```python
from build123d import *

# Parameters (mm, degrees)
F0_W      = 44.656470418
F0_H      = 33.8078811765
F1_DEPTH  = 16
F2_DEPTH  = 796
F3_DEPTH  = 196
F4_W      = 68.9578056335
F4_H      = 493.6993122101
F5_DEPTH  = 7
F6_DEPTH  = 9.7
F7_DEPTH  = 99.33
F8_DEPTH  = 99.33
F9_DEPTH  = 17.34
F10_DEPTH = 102.97
F11_W     = 35.2807044983
F11_H     = 492.0964837074
F12_DEPTH = 7
F13_DEPTH = 37.27
F14_DEPTH = 6.58
F15_DEPTH = 106.63
F16_DEPTH = 5.87
F17_DEPTH = 200
F18_DEPTH = 200
F19_DEPTH = 200
F20_DEPTH = 200
F21_DEPTH = 200
F22_DEPTH = 200
F23_DEPTH = 400
F24_DEPTH = 400
F25_DEPTH = 400
F26_DEPTH = 400
F27_DEPTH = 400
F28_DEPTH = 400
F29_DEPTH = 400
F30_DEPTH = 400
F31_DEPTH = 400
F32_DEPTH = 1000
F33_DEPTH = 1000
F34_DEPTH = 1000
F35_DEPTH = 1000
F36_DEPTH = 1000
F37_DEPTH = 1000
F38_R     = 3


with BuildPart() as f1:
    # F0 (on Front) → F1 (new body)
    with BuildSketch(Plane.XZ):
        with Locations((22.328235209, 16.9039405882)):
            Rectangle(F0_W, F0_H)
    extrude(amount=F1_DEPTH)

    # F2 (add): a face of the model
    f2_faces = [f1.faces().sort_by_distance(p)[0] for p in [
        (22.328235209, -8, 0),
    ]]
    extrude(f2_faces, amount=-F2_DEPTH)

    # F3 (add): a face of the model
    f3_faces = [f1.faces().sort_by_distance(p)[0] for p in [
        (0, -8, 398),
    ]]
    extrude(f3_faces, amount=-F3_DEPTH)

    # F4 (on face) → F5 (cut)
    with BuildSketch(Plane.XZ.offset(16)):
        with Locations((94.1769480705, 399.8196721077)):
            Rectangle(F4_W, F4_H)
    extrude(amount=-F5_DEPTH, mode=Mode.SUBTRACT)

    # F6 (cut): a face of the model
    f6_faces = [f1.faces().sort_by_distance(p)[0] for p in [
        (59.6980452538, -12.5, 399.8196721077),
    ]]
    extrude(f6_faces, amount=-F6_DEPTH, mode=Mode.SUBTRACT)

    # F7 (add): a face of the model
    f7_faces = [f1.faces().sort_by_distance(p)[0] for p in [
        (89.3269480705, -12.5, 646.6693282127),
    ]]
    extrude(f7_faces, amount=-F7_DEPTH)

    # F8 (cut): a face of the model
    f8_faces = [f1.faces().sort_by_distance(p)[0] for p in [
        (89.3269480705, -12.5, 646.6693282127),
    ]]
    extrude(f8_faces, amount=-F8_DEPTH, mode=Mode.SUBTRACT)

    # F9 (cut): a face of the model
    f9_faces = [f1.faces().sort_by_distance(p)[0] for p in [
        (128.6558508873, -12.5, 449.4846721077),
    ]]
    extrude(f9_faces, amount=-F9_DEPTH, mode=Mode.SUBTRACT)

    # F10 (cut): a face of the model
    f10_faces = [f1.faces().sort_by_distance(p)[0] for p in [
        (97.9969480705, -12.5, 152.9700160027),
    ]]
    extrude(f10_faces, amount=-F10_DEPTH, mode=Mode.SUBTRACT)

    # F11 (on face) → F12 (join)
    with BuildSketch(Plane.XZ.offset(9)):
        with Locations((91.7714834213, 432.6795041561)):
            Rectangle(F11_W, F11_H)
    extrude(amount=F12_DEPTH)

    # F13 (add): a face of the model
    f13_faces = [f1.faces().sort_by_distance(p)[0] for p in [
        (91.7714834213, -12.5, 678.7277460098),
    ]]
    extrude(f13_faces, amount=F13_DEPTH)

    # F14 (add): a face of the model
    f14_faces = [f1.faces().sort_by_distance(p)[0] for p in [
        (109.4118356705, -12.5, 451.3145041561),
    ]]
    extrude(f14_faces, amount=F14_DEPTH)

    # F15 (add): a face of the model
    f15_faces = [f1.faces().sort_by_distance(p)[0] for p in [
        (95.0614834213, -12.5, 186.6312623024),
    ]]
    extrude(f15_faces, amount=F15_DEPTH)

    # F16 (cut): a face of the model
    f16_faces = [f1.faces().sort_by_distance(p)[0] for p in [
        (74.1311311722, -12.5, 397.9995041561),
    ]]
    extrude(f16_faces, amount=-F16_DEPTH, mode=Mode.SUBTRACT)

    # F17 (add): a face of the model
    f17_faces = [f1.faces().sort_by_distance(p)[0] for p in [
        (196, -8, 398),
    ]]
    extrude(f17_faces, amount=F17_DEPTH)

    # F18 (cut): a face of the model
    f18_faces = [f1.faces().sort_by_distance(p)[0] for p in [
        (145.9958508873, -12.5, 397.9996721077),
    ]]
    extrude(f18_faces, amount=-F18_DEPTH, mode=Mode.SUBTRACT)

    # F19 (add): a face of the model
    f19_faces = [f1.faces().sort_by_distance(p)[0] for p in [
        (115.9918356705, -12.5, 397.9995041561),
    ]]
    extrude(f19_faces, amount=F19_DEPTH)

    # F20 (add): a face of the model
    f20_faces = [f1.faces().sort_by_distance(p)[0] for p in [
        (396, -8, 398),
    ]]
    extrude(f20_faces, amount=F20_DEPTH)

    # F21 (cut): a face of the model
    f21_faces = [f1.faces().sort_by_distance(p)[0] for p in [
        (345.9958508873, -12.5, 397.9996721077),
    ]]
    extrude(f21_faces, amount=-F21_DEPTH, mode=Mode.SUBTRACT)

    # F22 (add): a face of the model
    f22_faces = [f1.faces().sort_by_distance(p)[0] for p in [
        (315.9918356705, -12.5, 397.9995041561),
    ]]
    extrude(f22_faces, amount=F22_DEPTH)

    # F23 (add): a face of the model
    f23_faces = [f1.faces().sort_by_distance(p)[0] for p in [
        (596, -8, 398),
    ]]
    extrude(f23_faces, amount=F23_DEPTH)

    # F24 (cut): a face of the model
    f24_faces = [f1.faces().sort_by_distance(p)[0] for p in [
        (545.9958508873, -12.5, 397.9996721077),
    ]]
    extrude(f24_faces, amount=-F24_DEPTH, mode=Mode.SUBTRACT)

    # F25 (add): a face of the model
    f25_faces = [f1.faces().sort_by_distance(p)[0] for p in [
        (515.9918356705, -12.5, 397.9995041561),
    ]]
    extrude(f25_faces, amount=F25_DEPTH)

    # F26 (cut): a face of the model
    f26_faces = [f1.faces().sort_by_distance(p)[0] for p in [
        (497.9964834213, -12.5, 80.0012623024),
    ]]
    extrude(f26_faces, amount=-F26_DEPTH, mode=Mode.SUBTRACT)

    # F27 (add): a face of the model
    f27_faces = [f1.faces().sort_by_distance(p)[0] for p in [
        (497.9969480705, -12.5, 50.0000160027),
    ]]
    extrude(f27_faces, amount=F27_DEPTH)

    # F28 (cut): a face of the model
    f28_faces = [f1.faces().sort_by_distance(p)[0] for p in [
        (498, -8, 0),
    ]]
    extrude(f28_faces, amount=-F28_DEPTH, mode=Mode.SUBTRACT)

    # F29 (add): a face of the model
    f29_faces = [f1.faces().sort_by_distance(p)[0] for p in [
        (996, -8, 598),
    ]]
    extrude(f29_faces, amount=F29_DEPTH)

    # F30 (cut): a face of the model
    f30_faces = [f1.faces().sort_by_distance(p)[0] for p in [
        (945.9958508873, -12.5, 597.9996721077),
    ]]
    extrude(f30_faces, amount=-F30_DEPTH, mode=Mode.SUBTRACT)

    # F31 (add): a face of the model
    f31_faces = [f1.faces().sort_by_distance(p)[0] for p in [
        (915.9918356705, -12.5, 597.9995041561),
    ]]
    extrude(f31_faces, amount=F31_DEPTH)

    # F32 (cut): a face of the model
    f32_faces = [f1.faces().sort_by_distance(p)[0] for p in [
        (1315.9918356705, -12.5, 597.9995041561),
    ]]
    extrude(f32_faces, amount=-F32_DEPTH, mode=Mode.SUBTRACT)

    # F33 (add): a face of the model
    f33_faces = [f1.faces().sort_by_distance(p)[0] for p in [
        (1345.9958508873, -12.5, 597.9996721077),
    ]]
    extrude(f33_faces, amount=F33_DEPTH)

    # F34 (cut): a face of the model
    f34_faces = [f1.faces().sort_by_distance(p)[0] for p in [
        (1396, -8, 598),
    ]]
    extrude(f34_faces, amount=-F34_DEPTH, mode=Mode.SUBTRACT)

    # F35 (add): a face of the model
    f35_faces = [f1.faces().sort_by_distance(p)[0] for p in [
        (198, -8, 796),
    ]]
    extrude(f35_faces, amount=F35_DEPTH)

    # F36 (cut): a face of the model
    f36_faces = [f1.faces().sort_by_distance(p)[0] for p in [
        (197.9969480705, -12.5, 745.9993282127),
    ]]
    extrude(f36_faces, amount=-F36_DEPTH, mode=Mode.SUBTRACT)

    # F37 (add): a face of the model
    f37_faces = [f1.faces().sort_by_distance(p)[0] for p in [
        (197.9964834213, -12.5, 715.9977460098),
    ]]
    extrude(f37_faces, amount=F37_DEPTH)

    # F38
    f38_edges = [f1.edges().sort_by_distance(p)[0] for p in [
        (80.001131, -16, 1097.999504),
        (197.996483, -16, 1715.997746),
        (315.991836, -16, 1097.999504),
        (197.996483, -16, 480.001262),
        (0, -16, 1098),
        (198, -16, 400),
        (396, -16, 1098),
        (198, -16, 1796),
        (345.995851, -16, 1097.999672),
        (197.996948, -16, 450.000016),
        (49.998045, -16, 1097.999672),
        (197.996948, -16, 1745.999328),
    ]]
    fillet(f38_edges, radius=F38_R)


solid = f1.part
```
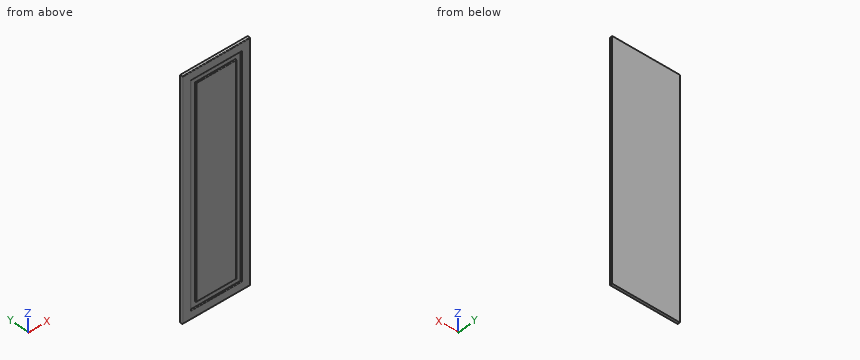
For this review, take the finished solid that the model builds, in its own axes (mm). Coordinates: 2 decimals unless noted, no trailing zeros. Write each loop counter-clockwise with the first axis right and the second up, starting at its lowest first coordinate (ties: lowest second). Pieces come first, ordered by that corner, then holes. Notation, with made-up numbers: (10.25, 83.5) - (60.25, 83.5) arc R15 cw to (60.25, 93.5) - close; hole circle Ø9 at (3, 46). An arc over 180 degrees is marked (long way). Answer in a Markdown table with one row per item. Add a question column.
Q1. We need section A-A, the plane x = 97.5. State the section outline as (y, z) points.
Q2. We need section B-B, the plane z = 1352.5. State the section outline as (x, y) points.
Q3. For probe 1 along Z at (x, y) = (294, -10.75); probe 2 along X at (y, z) = (-11.5, 1620.5); probe 3 along Z at (x, y) = (144, -15), list the stretches that pass through material, from the lowest coordinate up.
Answer list:
| question | item | result |
|---|---|---|
| 1 | outline | (-16, 403) arc R3 ccw to (-13, 400) - (0, 400) - (0, 1796) - (-13, 1796) arc R3 ccw to (-16, 1793) - (-16, 1749) arc R3 ccw to (-13, 1746) - (-9, 1746) - (-9, 1716) - (-13, 1716) arc R3 ccw to (-16, 1713) - (-16, 483) arc R3 ccw to (-13, 480) - (-9, 480) - (-9, 450) - (-13, 450) arc R3 ccw to (-16, 447) - close |
| 2 | outline | (0, -13) arc R3 ccw to (3, -16) - (47, -16) arc R3 ccw to (50, -13) - (50, -9) - (80, -9) - (80, -13) arc R3 ccw to (83, -16) - (312.99, -16) arc R3 ccw to (315.99, -13) - (315.99, -9) - (346, -9) - (346, -13) arc R3 ccw to (349, -16) - (393, -16) arc R3 ccw to (396, -13) - (396, 0) - (0, 0) - close |
| 3 | probe 1 | z = 400 to 450, 480 to 1716, 1746 to 1796 |
| 3 | probe 2 | x = 0 to 50, 80 to 315.99, 346 to 396 |
| 3 | probe 3 | z = 400.76 to 449.24, 480.77 to 1715.23, 1746.76 to 1795.24 |
